from build123d import *

# Parameters (mm, degrees)
F0_W     = 50
F0_H     = 110
F1_DEPTH = 60
F2_W     = 30
F2_H     = 16.95089
F2_W_2   = 10
F2_H_2   = 10
F3_DEPTH = 50.001
F4_W     = 20
F4_H     = 45
F5_DEPTH = 10


with BuildPart() as f1:
    # F0 (on Top) → F1 (new body)
    with BuildSketch(Plane.XY):
        Rectangle(F0_W, F0_H)
    extrude(amount=F1_DEPTH)

    # F2 (on face) → F3 (cut, through all)
    with BuildSketch(Plane.YZ.offset(25)):
        with Locations((30, 31.524555)):
            Rectangle(F2_W, F2_H)
        with Locations((50, 55)):
            Rectangle(F2_W_2, F2_H_2)
        with Locations((10, 55)):
            Rectangle(F2_W_2, F2_H_2)
        Polygon((5, 50), (5, 60), (-55, 60), (-55, 23.04911), (5, 23.04911), align=None)
    extrude(amount=-F3_DEPTH, mode=Mode.SUBTRACT)

    # F4 (on face) → F5 (cut)
    with BuildSketch(Plane.XY.offset(23.04911)):
        with Locations((0, -17.5)):
            Rectangle(F4_W, F4_H)
    extrude(amount=-F5_DEPTH, mode=Mode.SUBTRACT)


solid = f1.part
Design review of the part built by this model. Coordinates are the model's own, in mm. A direction names the side the tool comes from. Give positions to 0.01 mm unless a question says otherwise; leave off trailing zeros. Order: outer loops, then holes, each group sorted by start corner. A loop starts at its lowest first (then second) coordinate and runs counter-clockwise, first axis right, second up. Notation, with made-up numbers: (52.5, 82) - (95.5, 82) arc R19 cw to (95.5, 106) - close; hole circle Ø6 at (52.5, 37). An arc over 180 degrees is marked (long way). Write item = value, one per line. Start each with the question number.
Q1. To check wall thickness, follow L1, parallel to Z at x = 9.5, y = 35; L2, parallel to Y at x = -16, z = 30.5; L3, parallel to X at y = -11.5, z = 19. State the ranges of each line that lie inside material, in increasing order. Write a range as from..to.
Q2. Mouldability with a two-part tool opening along Z and no side actions: class faces 5 (the face through (10, -18, 18)), 6 (the face through (0, 45, 31)), 7 (the face through (0, 30, 60)) as released by +Z, released by -Z, zero draft, split by the parting line, or undercut.
Q3. We need section D-D on y = -11. State the section outline as (x, z) points, plus the area to 3 significant figures.
Q4. Clearance check with flat-ended pins moving along their axes: pin 1 Ø10 at (x, z) = (10.5, 36.5) entering from -Y; pin 2 Ø3 at (x, y) = (4, 10) entering from +Z; pin 3 Ø6 at (x, z) = (-9.5, 54) entering from +Y. State where each tip first meets the part, or that it passes through.
Q5. We need section C-C on x = -16. State the section outline as (y, z) points, plus the area to 3 significant figures.
Q6. We need section B-B on y = 18.5. State the section outline as (x, z) points, plus the area to 3 significant figures.
Q7. Tool access review of faces 1 (the face through (0, -17, 13.049)), 2 (the face through (11, -25, 23.049)), 3 (the face through (0, 30, 23.049)), 4 (the face through (0, 45, 55)): name each direction out of +Z, -Z, +X, -X, +Y, -Y from which nothing blocks a thin tool from reaching the whole face with its end or side.
Q8. We need section A-A on z = 19.5. State the section outline as (x, y) points, plus the area to 3 significant figures.
Working result:
q1.L1 = 0..23.05, 40..60
q1.L2 = 5..15, 45..55
q1.L3 = -25..-10, 10..25
q2.face_5 = zero draft
q2.face_6 = undercut
q2.face_7 = released by +Z
q3.outline = (-25, 0) - (25, 0) - (25, 23.05) - (10, 23.05) - (10, 13.05) - (-10, 13.05) - (-10, 23.05) - (-25, 23.05) - close
q3.area = 952 mm²
q4.pin_1 = 5
q4.pin_2 = 50
q4.pin_3 = 45
q5.outline = (-55, 0) - (55, 0) - (55, 50) - (45, 50) - (45, 60) - (15, 60) - (15, 50) - (5, 50) - (5, 23.05) - (-55, 23.05) - close; hole (15, 23.05) - (45, 23.05) - (45, 40) - (15, 40) - close
q5.area = 3,670 mm²
q6.outline = (-25, 0) - (25, 0) - (25, 23.05) - (-25, 23.05) - close; (-25, 40) - (25, 40) - (25, 60) - (-25, 60) - close
q6.area = 2,150 mm²
q7.face_1 = +Z
q7.face_2 = +Z, +X, -X, -Y
q7.face_3 = +X, -X
q7.face_4 = +Z, +X, -X, +Y
q8.outline = (-25, -55) - (25, -55) - (25, 55) - (-25, 55) - close; hole (-10, -40) - (10, -40) - (10, 5) - (-10, 5) - close
q8.area = 4,600 mm²
